Geometry: final body of the model. Coordinates: model frame, mm. Face numbers are marked on the shaded views. A direction names the side the tool comes from. Give positions to 0.01 mm unless a question says otherwise; leave off trailing zeros. Write each loop counter-clockwise with the first axis right and the second up, starting at its lowest first coordinate (ties: lowest second). Pieces come first, ordered by that corner, then holes.
Q1. Section B-B (x = 82.46). Return the cut outline in (y, z).
Q2. Section C-C (y = 3.25). Return the cut outline in (x, z).
Q3. Section D-D (x = 73.5). Return the cut outline in (y, z).
Q4. Pin query (flat end, axial travel): pin 1 Ø4 at (y, z) = (2.5, -12.5) entering from +X; pin 2 Ø1 at (x, y) = (18.5, 6) entering from -Z; pin 3 Ø5.5 at (x, z) = (82.46, -51.46) entering from +Y; pin 4 Ø4.5 at (y, z) = (7.5, -49.5) entering from -X. Return the tip coordinate at first contact, or that it passes through.
Q5. Mould query, pull axis X, two halves, no side actions, for the marked faces 1 and 2. Classes: +X half, -X half, draft (parallel to the pull), parting line (faces both ways), or undercut.
Q6. Section A-A (z = -2.54). Return the cut outline in (x, y).
Q7. Line query: line 1 (Z direction, x = 82.46, y = 0.85); line 2 (Z direction, x = 15.5, y = 2.5); line 3 (X direction, y = 1.5, z = -51). Output: solid intervals per line, ascending.
Q8. Reachability of the marked faces 3, 4, 5 and 6 from +Z, -Z, +X, -X, +Y, -Y: full face, straight path, thin tool, end or side. Return the list, or none.
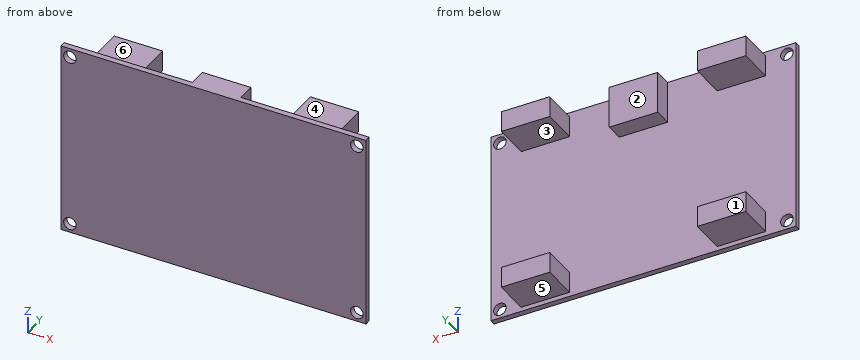
from build123d import *

# Parameters (mm, degrees)
SKETCH7_W                  = 85
SKETCH7_H                  = 54
BOSS_EXTRUDE2_DEPTH        = 1.6
F_3_5_3_5_DIAMETER_HOLE1_D = 3.5
SKETCH14_W                 = 13.5
SKETCH14_H                 = 5.8
BOSS_EXTRUDE3_DEPTH        = 10
LPATTERN1_COUNT            = 2
LPATTERN1_PITCH            = 54.6
LPATTERN1_COUNT_DIR2       = 2
LPATTERN1_PITCH_DIR2       = 45.8
SKETCH15_W                 = 13.5
SKETCH15_H                 = 11.7
BOSS_EXTRUDE4_DEPTH        = 5


with BuildPart() as part:
    # Sketch7 → Boss-Extrude2 (new body)
    with BuildSketch(Plane(origin=(0, 0, 0), x_dir=(1, 0, 0), z_dir=(0, 1, 0))):
        with Locations((42.5, 27)):
            Rectangle(SKETCH7_W, SKETCH7_H)
    extrude(amount=BOSS_EXTRUDE2_DEPTH)

    # Ø3.5 (3.5) Diameter Hole1 (through all)
    with Locations(Plane(origin=(0, 1.6, 0), x_dir=(-1, 0, 0), z_dir=(0, 1, 0))):
        with Locations((-2.54, -2.54), (-2.54, -51.46), (-82.46, -51.46), (-82.46, -2.54)):
            Hole(F_3_5_3_5_DIAMETER_HOLE1_D / 2)

    # Sketch14 → Boss-Extrude3 (add)
    with BuildSketch(Plane(origin=(0, 1.6, 0), x_dir=(1, 0, 0), z_dir=(0, 1, 0))):
        with Locations((15.2, 49.9)):
            Rectangle(SKETCH14_W, SKETCH14_H)
    boss_extrude3 = extrude(amount=BOSS_EXTRUDE3_DEPTH)

    # LPattern1: Boss-Extrude3 2 × 2
    with Locations(*[(i * LPATTERN1_PITCH, 0, j * LPATTERN1_PITCH_DIR2) for i in range(LPATTERN1_COUNT) for j in range(LPATTERN1_COUNT_DIR2) if (i, j) != (0, 0)]):
        add(boss_extrude3)

    # Sketch15 → Boss-Extrude4 (add)
    with BuildSketch(Plane(origin=(0, 1.6, 0), x_dir=(1, 0, 0), z_dir=(0, 1, 0))):
        with Locations((42.5, 5.85)):
            Rectangle(SKETCH15_W, SKETCH15_H)
    extrude(amount=BOSS_EXTRUDE4_DEPTH)


solid = part.part
Computed:
1. outline: (0, -54) - (1.6, -54) - (1.6, -53.21) - (0, -53.21) - close; (0, -49.71) - (1.6, -49.71) - (1.6, -4.29) - (0, -4.29) - close; (0, -0.79) - (1.6, -0.79) - (1.6, 0) - (0, 0) - close
2. outline: (8.45, -52.8) - (21.95, -52.8) - (21.95, -47) - (8.45, -47) - close; (8.45, -7) - (21.95, -7) - (21.95, -1.2) - (8.45, -1.2) - close; (35.75, -11.7) - (49.25, -11.7) - (49.25, 0) - (35.75, 0) - close; (63.05, -52.8) - (76.55, -52.8) - (76.55, -47) - (63.05, -47) - close; (63.05, -7) - (76.55, -7) - (76.55, -1.2) - (63.05, -1.2) - close
3. outline: (0, -54) - (1.6, -54) - (1.6, -52.8) - (11.6, -52.8) - (11.6, -47) - (1.6, -47) - (1.6, -7) - (11.6, -7) - (11.6, -1.2) - (1.6, -1.2) - (1.6, 0) - (0, 0) - close
4. pin 1: stops at x = 85
4. pin 2: stops at z = -52.8
4. pin 3: stops at y = 1.6
4. pin 4: stops at x = 8.45
5. face 1: draft
5. face 2: undercut
6. outline: (0, 0) - (0.79, 0) - (0.79, 1.6) - (0, 1.6) - close; (4.29, 0) - (80.71, 0) - (80.71, 1.6) - (76.55, 1.6) - (76.55, 11.6) - (63.05, 11.6) - (63.05, 1.6) - (49.25, 1.6) - (49.25, 6.6) - (35.75, 6.6) - (35.75, 1.6) - (21.95, 1.6) - (21.95, 11.6) - (8.45, 11.6) - (8.45, 1.6) - (4.29, 1.6) - close; (84.21, 0) - (85, 0) - (85, 1.6) - (84.21, 1.6) - close
7. line 1: z = -54 to -53.21, -49.71 to -4.29, -0.79 to 0
7. line 2: z = -52.8 to -47, -7 to -1.2
7. line 3: x = 0 to 0.85, 4.23 to 80.77, 84.15 to 85
8. face 3: +X, +Y
8. face 4: +Z, +X, +Y
8. face 5: -Z, +X, -X, +Y
8. face 6: +Z, -X, +Y
